For this review, use the dimensioned drawing (mm, ordinates from the lowest corner) and the shaded views. Round coordinates to 2 decimals unless told otherwise and drop trailing zeros. Write each loop counter-clockwise with the first axis right and the second up, starting at its lowest first coordinate (ties: lowest second). Pieces come first, ordered by that corner, then holes.
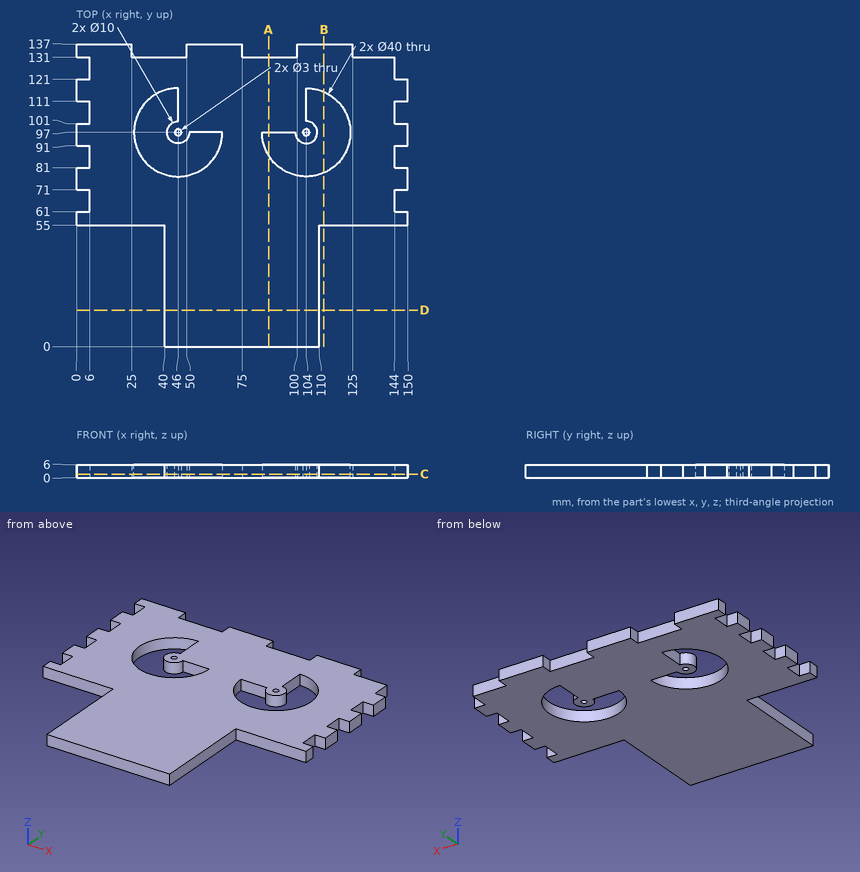
(1) We need section C-C, the plane z = 1.65. State how many separate pieces and enclosed holes the cut face has, and give its area (3 significant figures).
Geometry check:
separate pieces: 1
enclosed holes: 4
area: 13,400 mm2
(2) We need section A-A, the plane x = 87. Give the boundary of the cut face in (y, z).
Geometry check:
outline: (0, 0) - (86.46, 0) - (86.46, 6) - (0, 6) - close; (97, 0) - (131, 0) - (131, 6) - (97, 6) - close
(3) For pin 1 Ø3 at (x, z) = (147.5, 4.5) entering from -Y; pin 2 Ø1 at (y, z) = (85.5, 4.5) entering from -X; pin 3 Ø1.8 at (y, z) = (108.5, 4.5) entering from +X, all flat-tipped, find the tip position at first contact; note any pin that passes through.
Geometry check:
pin 1: stops at y = 55
pin 2: stops at x = 6
pin 3: stops at x = 144
(4) We need section D-D, the plane y = 16.5. Give the boundary of the cut face in (x, z), and give its area (3 significant figures).
Geometry check:
outline: (40, 0) - (110, 0) - (110, 6) - (40, 6) - close
area: 420 mm2
(5) We need section B-B, the plane x = 112. Give the boundary of the cut face in (y, z).
Geometry check:
outline: (55, 0) - (78.67, 0) - (78.67, 6) - (55, 6) - close; (115.33, 0) - (137, 0) - (137, 6) - (115.33, 6) - close
(6) For line 1 along X through (y, z) = (83.5, 1.65); line 2 along X through (y, z) = (90.5, 1.25); line 3 along X through (y, z) = (9, 1.7), list the stretches that pass through material, from the lowest coordinate up.
Geometry check:
line 1: x = 6 to 31.24, 60.76 to 89.24, 118.76 to 144
line 2: x = 6 to 27.09, 64.91 to 85.09, 122.91 to 144
line 3: x = 40 to 110
